The figure shows three views and two pictorial views of one solid part (mm, origin at its lowest corner). Answer the questions. Round coordinates to 2 decimals unless told otherwise and drop trailing zeros. Write each loop counter-clockwise with the first axis right and the second up, starting at its lowest first coordinate (ties: lowest second). Pieces come first, ordered by that corner, then holes.
Item 1: Find section A-A on x = 12.5. Give the vertices of the cut face in (y, z) (1 decimal), then the cut area to 3 significant figures.
Item 2: Find the intervals of material crossed by probe 1 along Y at (x, z) = (12, 2.8) (1 decimal); probe 2 along X at (y, z) = (9.5, 0.6); probe 3 along Y at (x, z) = (38.1, 3.25) (1 decimal), in increasing order.
Item 3: Find section B-B on y = 7. Give the vertices of the cut face in (x, z).
Item 4: This flat-tipped pin is pushed along its axis until it touches: pin 1 (2.5 mm diameter, centred on y = 8, z = 1, fed in from +X). Where does it stop, or does it pass through?
Item 5: Find section D-D on x = 45. Give the vertices of the cut face in (y, z) (1 decimal).
Item 6: Find section C-C on z = 2.65. Give the vertices of the cut face in (x, y) (1 decimal), then the cut area to 3 significant figures.
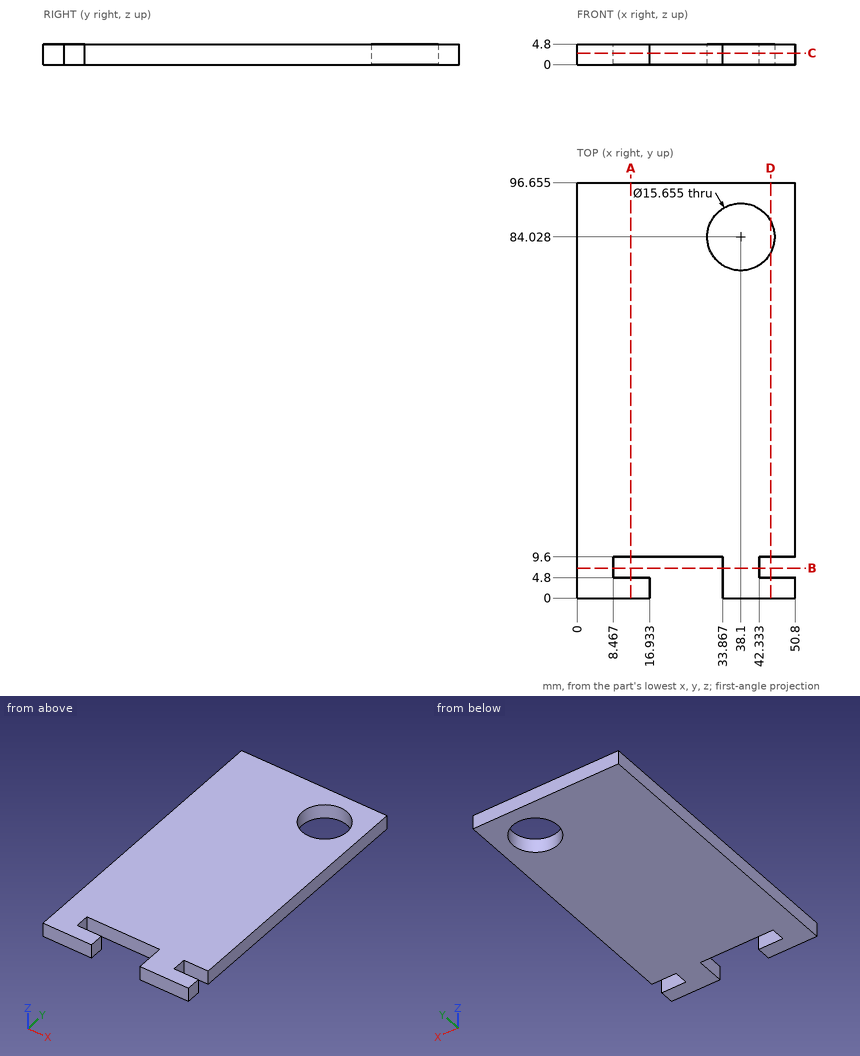
Check values:
1. outline: (0, 0) - (4.8, 0) - (4.8, 4.8) - (0, 4.8) - close; (9.6, 0) - (96.7, 0) - (96.7, 4.8) - (9.6, 4.8) - close
1. area: 441 mm2
2. probe 1: y = 0 to 4.8, 9.6 to 96.7
2. probe 2: x = 0 to 8.47, 33.87 to 42.33
2. probe 3: y = 0 to 76.2, 91.9 to 96.7
3. outline: (0, 0) - (8.47, 0) - (8.47, 4.8) - (0, 4.8) - close; (33.87, 0) - (42.33, 0) - (42.33, 4.8) - (33.87, 4.8) - close
4. pin 1: stops at x = 42.33
5. outline: (0, 0) - (4.8, 0) - (4.8, 4.8) - (0, 4.8) - close; (9.6, 0) - (80.3, 0) - (80.3, 4.8) - (9.6, 4.8) - close; (87.7, 0) - (96.7, 0) - (96.7, 4.8) - (87.7, 4.8) - close
6. outline: (0, 0) - (16.9, 0) - (16.9, 4.8) - (8.5, 4.8) - (8.5, 9.6) - (33.9, 9.6) - (33.9, 0) - (50.8, 0) - (50.8, 4.8) - (42.3, 4.8) - (42.3, 9.6) - (50.8, 9.6) - (50.8, 96.7) - (0, 96.7) - close; hole circle Ø15.7 at (38.1, 84)
6. area: 4,470 mm2
